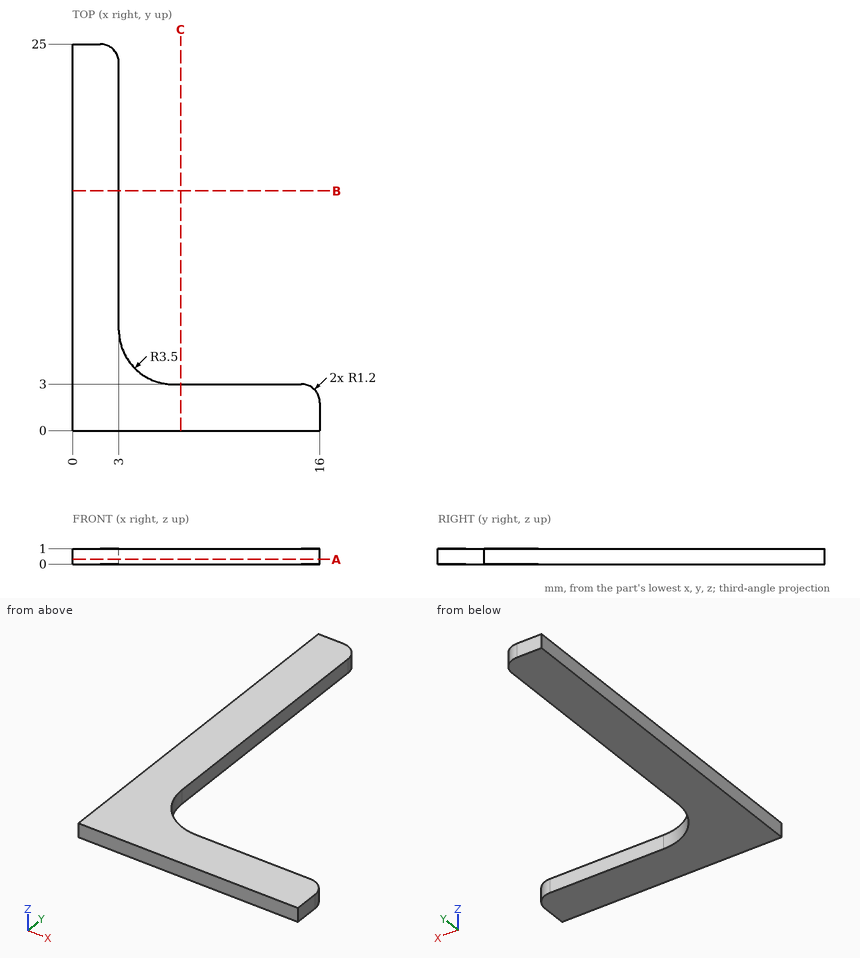
Job drawing, mm, ordinate dimensions from the low corner. One solid piece. Coordinates: 2 decimals unless noted, no trailing zeros. Write each loop counter-clockwise with the first axis right and the second up, starting at its lowest first coordinate (ties: lowest second). Pieces come first, ordered by that corner, then holes. Notation, with made-up numbers: M 11.5,-33.5 L 58.5,-33.5 A25 cw 58.5,-14.5 Z; hole C -20.5,89 d5. An arc over 180 degrees is marked long. Answer as a JSON object with one key per item and string values. Group by question number.
1) Wall check: line 1 (X direction, y = 7.5, z = 0.5); line 2 (Y direction, x = 2.75, z = 0.4). Give the ranges that are in metal, low to high. Write a range as from..to.
2) Saw through at A-A (z = 0.3). Write the cut outline in (x, y).
3) Saw through at B-B (y = 15.5). Write the cut outline in (x, z), plus the area to 3 significant figures.
Values follow:
{
 "1": {"line 1": "x = 0..3", "line 2": "y = 0..24.53"},
 "2": {"outline": "M 0,0 L 16,0 L 16,1.8 A1.2 ccw 14.8,3 L 6.5,3 A3.5 cw 3,6.5 L 3,23.8 A1.2 ccw 1.8,25 L 0,25 Z"},
 "3": {"outline": "M 0,0 L 3,0 L 3,1 L 0,1 Z", "area": "3.00 mm2"}
}
